Work out the finished part from the listing and answer in its coordinate system (mm). Give positions to 0.01 mm unless a question says otherwise; leave off trailing zeros. Loops run counter-clockwise (first coordinate to the right, second up) from the corner with the lowest first, then second, coordinate; pieces in that order, holes last.
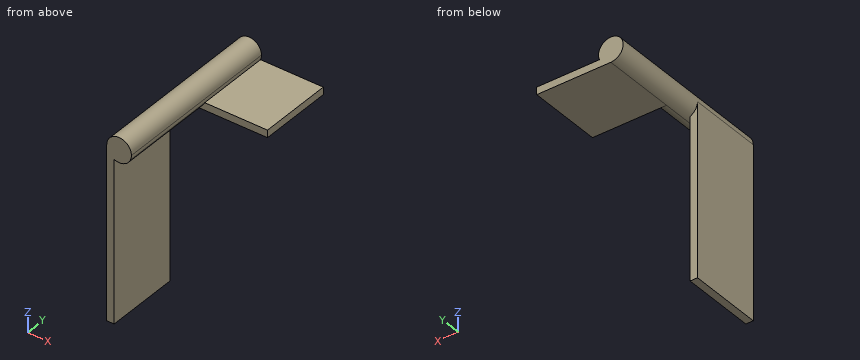
```python
from build123d import *

# Parameters (mm, degrees)
F1_DEPTH = 70
F2_DEPTH = 30
F4_DEPTH = 30


# Not quite as in the source:
# - a feature names something its author has since deleted; it is built from what else it names


with BuildPart() as f1:
    # F0 (on Front) → F1 (new body)
    with BuildSketch(Plane.XZ):
        with BuildLine():
            ThreePointArc((4.582575695, -2), (4.8945315647, -1.0215482184), (5, 0))
            ThreePointArc((5, 0), (-3.5355339059, 3.5355339059), (0, -5))
            Line((0, -5), (0, -2))
            Line((0, -2), (4.582575695, -2))
        make_face()
        with BuildLine():
            Line((0, -2), (0, -5))
            ThreePointArc((0, -5), (2.7386127875, -4.1833001327), (4.582575695, -2))
            Line((4.582575695, -2), (0, -2))
        make_face()
    extrude(amount=F1_DEPTH)

    # F0 (on Front) → F2 (join)
    with BuildSketch(Plane.XZ):
        with BuildLine():
            ThreePointArc((4.582575695, -2), (2.7386127875, -4.1833001327), (0, -5))
            Line((0, -5), (30, -5))
            Line((30, -5), (30, -2))
            Line((30, -2), (4.582575695, -2))
        make_face()
    extrude(amount=F2_DEPTH)

    # F3 (on face) → F4 (join)
    with BuildSketch(Plane.XZ.offset(70)):
        with BuildLine():
            Line((-2, -70), (-2, -4.582575695))
            ThreePointArc((-2, -4.582575695), (-4.1833001327, -2.7386127875), (-5, 0))
            Line((-5, 0), (-5, -70))
            Line((-5, -70), (-2, -70))
        make_face()
    extrude(amount=-F4_DEPTH)


solid = f1.part
```
Q1. Section A-A on y = -43 is taken. Give the vertices of the cut face in (x, z).
Q2. Section B-B on x = 2 is taken. Give the vertices of the cut face in (y, z), plus the area to 3 significant figures.
Q3. Given pin 1 (8 mm diameter, centred on x = 3, y = -48.5, fed in from -Z); pin 2 (0.9 mm diameter, centred on x = 18.5, z = -3, fed in from -Y); pin 3 (8 mm diameter, centred on y = -40.5, z = -6, fed in from +X); pin 4 (1 mm diameter, centred on y = -38.5, z = -12.5, fed in from +X), each flat-ended and moving along its own axis, determine where each tip first touches the part or whether it passes through.
Q4. Section D-D on y = -11.5 is taken. Give the vertices of the cut face in (x, z), plus the area to 3 significant figures.
Q5. Consider line 1 along X through (y, z) = (-56, -16); line 2 along Y through (x, z) = (17, -4). Determine where each line is inside the solid, lowest interval first.
Q6. Section C-C on z = -22 is taken. Give the vertices of the cut face in (x, y), plus the area to 3 significant figures.
Check result:
1. outline: (-5, -70) - (-2, -70) - (-2, -4.58) arc R5 ccw (long way) to (-5, 0) - close
2. outline: (-70, -4.58) - (-30, -4.58) - (-30, -5) - (0, -5) - (0, 4.58) - (-70, 4.58) - close
2. area: 654 mm2
3. pin 1: stops at z = -5
3. pin 2: stops at y = -30
3. pin 3: stops at x = 4.58
3. pin 4: passes through
4. outline: (0, -5) - (30, -5) - (30, -2) - (4.58, -2) arc R5 ccw (long way) to start
4. area: 159 mm2
5. line 1: x = -5 to -2
5. line 2: y = -30 to 0
6. outline: (-5, -70) - (-2, -70) - (-2, -40) - (-5, -40) - close
6. area: 90.0 mm2
